Work out the finished part from the listing and answer in its coordinate system (mm). Face numbers are marked on the shaded views. A direction names the side the tool comes from. Give positions to 0.01 mm unless a question says otherwise; leave off trailing zeros. Loops run counter-clockwise (first coordinate to the right, second up) from the corner with the lowest first, then second, coordinate; pieces in that order, holes last. Notation, with made-up numbers: M 45,-22 L 93,-22 A29 cw 93,-1 Z; hole C 51,46 d2. An arc over 180 degrees is marked long. Write item = value, one per line. Start each with the question number.
1. Flat-ended cylindrical pins translate along their axes: pin 1 Ø2 at (x, z) = (9.5, 4) entering from +Y; pin 2 Ø1 at (x, z) = (17.5, 1) entering from +Y; pin 3 Ø1.5 at (x, z) = (6, 3.5) entering from -Y; pin 4 Ø1.5 at (y, z) = (51, 1) entering from +X. Find the tip coordinate at first contact, or state that the pin passes through.
2. Section B-B on y = 23.5 is taken. Determine the outline of the cut face in (x, z), plus the area to 3 significant figures.
3. Section A-A on z = 4.1 is taken. Determine the outline of the cut face in (x, y) (3 decimals), plus the area to 3 significant figures.
4. Consider L1, parallel to X at y = 8, z = 4.25; L2, parallel to X at y = 29.5, z = 4.5; L3, parallel to Y at x = 12.5, z = 4.85. Determine where each line is inside the solid, lowest interval first. Write a range as [from, to].
5. Section C-C on x = 4.75 is taken. Determine the outline of the cut face in (y, z), plus the area to 3 significant figures.
6. For the marked faces 1 and 2, determine the directions among +Z, -Z, +X, -X, +Y, -Y from which every point of the face is accessible in a straight line to the end or side of a thin tool.
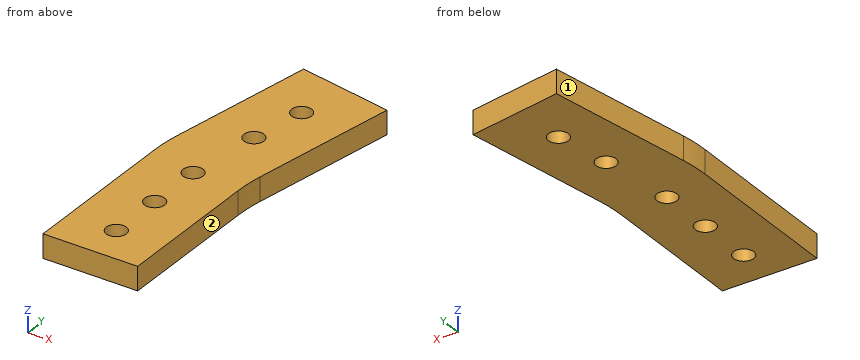
```python
from build123d import *

# Parameters (mm, degrees)
SKETCH_1_R      = 2.125
EXTRUDE_1_DEPTH = 5
FILLET_1_R      = 35


with BuildPart() as part:
    # 草图1 → 凸台-拉伸1 (new body)
    with BuildSketch(Plane.XY):
        Polygon((0, 0), (0, 38), (6.077686218, 72.468271355), (26.077686218, 68.941731741), (20, 34.473460386), (20, 0), align=None)
        with Locations((10, 32.118365096)):
            Circle(SKETCH_1_R, mode=Mode.SUBTRACT)
        with Locations((10, 20.118365096)):
            Circle(SKETCH_1_R, mode=Mode.SUBTRACT)
        with Locations((10, 8.118365096)):
            Circle(SKETCH_1_R, mode=Mode.SUBTRACT)
        with Locations((14.167556264, 59.872116265)):
            Circle(SKETCH_1_R, mode=Mode.SUBTRACT)
        with Locations((12.083778132, 48.054423229)):
            Circle(SKETCH_1_R, mode=Mode.SUBTRACT)
    extrude(amount=EXTRUDE_1_DEPTH)

    # 圆角1
    fillet_1_edges = [part.edges().sort_by_distance(p)[0] for p in [
        (0, 38, 2.5),
        (20, 34.473460386, 2.5),
    ]]
    fillet(fillet_1_edges, radius=FILLET_1_R)


solid = part.part
```
Verdict:
q1.pin_1 = 72.04
q1.pin_2 = 70.54
q1.pin_3 = 0
q1.pin_4 = 23.05
q2.outline = M 0,0 L 20,0 L 20,5 L 0,5 Z
q2.area = 100 mm2
q3.outline = M 0,0 L 20,0 L 20,31.411 A35 cw 20.532,37.489 L 26.078,68.942 L 6.078,72.468 L 0.532,41.016 A35 ccw 0,34.938 Z; hole C 10,8.118 d4.25; hole C 10,20.118 d4.25; hole C 10,32.118 d4.25; hole C 12.084,48.054 d4.25; hole C 14.168,59.872 d4.25
q3.area = 1,360 mm2
q4.L1 = [0, 7.88], [12.12, 20]
q4.L2 = [0, 20]
q4.L3 = [0, 45.97], [50.14, 58.55], [61.19, 71.34]
q5.outline = M 0,0 L 64.94,0 L 64.94,5 L 0,5 Z
q5.area = 325 mm2
q6.face_1 = +Z, -Z, -X, +Y
q6.face_2 = +Z, -Z, +X, -Y
